Source: CAD feature listing. Evaluate the final solid. Frame: model axes, mm. Coordinates: 2 decimals unless noted, no trailing zeros. Order: outer loops, then holes, each group sorted by start corner. A loop starts at its lowest first (then second) coordinate and runs counter-clockwise, first axis right, second up.
Autodesk Inventor part; units mm, degrees
ref_plane "YZ Plane" through (0, 0, 0) normal (1, 0, 0) x (0, 1, 0)
ref_plane "XZ Plane" through (0, 0, 0) normal (0, 1, 0) x (-1, 0, 0)
ref_plane "XY Plane" through (0, 0, 0) normal (0, 0, 1) x (1, 0, 0)
sketch "Sketch1" plane through (0, 0, 0) normal (0, 0, 1) x (1, 0, 0)
  circle A0 centre (78.7027, 64.253) radius 50.8 construction
  circle A1 centre (-78.7027, -64.253) radius 50.8 construction
  circle A2 centre (0, 0) radius 50.8 construction
  line L0 (-39.3513, -32.1265) -> (39.3513, 32.1265) construction
  line L1 (78.7027, 64.253) -> (-78.7027, -64.253) construction
  line L2 (-3.7208, 6.6498) -> (-3.7208, 50.6636) construction
  line L3 (-410.4212, -115.053) -> (454.9708, -115.053) construction
  circle A3 centre (140.9799, -57.903) radius 57.15 construction
  circle A4 centre (78.7027, 64.253) radius 14.2621
  circle A5 centre (-78.7027, -64.253) radius 14.2621
  circle A6 centre (-3.7208, 6.6498) radius 57.15 construction
  circle A7 centre (-78.7027, -64.253) radius 30.1371 construction
  circle A8 centre (78.7027, 64.253) radius 30.1371 construction
  circle A9 centre (-45.946, 108.8074) radius 14.2621
  line L4 (-45.946, 108.8074) -> (78.7027, 64.253) construction
  circle A10 centre (78.7027, 64.253) radius 14.2875 construction
  circle A11 centre (-78.7027, -64.253) radius 14.2875 construction
  circle A12 centre (-70.3302, 67.854) radius 14.2621
  line L5 (-78.7027, -64.253) -> (-70.3302, 67.854) construction
  circle A13 centre (-70.3302, 67.854) radius 23.8316 construction
  circle A14 centre (-45.946, 108.8074) radius 23.8316 construction
  line L6 (20.6869, 58.3256) -> (65.8317, 37.0027)
  line L7 (-49.1354, -58.4201) -> (-59.7901, -4.4114)
  arc A15 (20.6869, 58.3256) -> (-59.7901, -4.4114) centre (-3.7208, 6.6498) ccw
  line L8 (-201.842, 171.7522) -> (-176.8279, 167.3416)
  line L9 (-176.8279, 167.3416) -> (-203.2918, 17.2569) construction
  line L10 (-203.2918, 17.2569) -> (-228.306, 21.6675) construction
  line L11 (-228.306, 21.6675) -> (-201.842, 171.7522) construction
  line L12 (-247.3095, -86.1068) -> (28.2095, -134.6882) construction
  line L13 (-202.9446, 165.4987) -> (190.461, 96.1307) construction
  line L14 (-202.9446, 165.4987) -> (-247.3095, -86.1068) construction
  circle A16 centre (-145.4023, 107.8713) radius 31.75 construction
  line L15 (-71.8375, 44.0702) -> (-75.4896, -13.5547) construction
  circle A17 centre (21.8974, 84.5575) radius 9.525 construction
  line L16 (-189.3349, 169.5469) -> (-215.7989, 19.4622) construction
  line L17 (-192.0916, 153.9131) -> (-213.0422, 35.096) construction
  circle A18 centre (-145.4023, 107.8713) radius 17.4625 construction
  circle A19 centre (-145.4023, 107.8713) radius 9.525
  circle A20 centre (-45.946, 108.8074) radius 30.1816 construction
  line L18 (-201.842, 171.7522) -> (-228.306, 21.6675)
  arc A21 (65.8317, 37.0027) -> (86.8534, 93.267) centre (78.7027, 64.253) ccw
  arc A22 (-108.4816, -68.8852) -> (-49.1354, -58.4201) centre (-78.7027, -64.253) ccw
  line L19 (-145.4023, 107.8713) -> (-128.993, 113.8438) construction
  line L20 (-111.0918, 120.3593) -> (-179.7129, 95.3833) construction
  circle A23 centre (-179.7129, 95.3833) radius 4.7625 construction
  line L21 (0, 0) -> (-3.7208, 6.6498) construction
  circle A24 centre (78.7027, 64.253) radius 28.6512 construction
  line L22 (66.1835, 38.4817) -> (-52.1778, 95.9789) construction
  line L23 (85.3564, 92.1209) -> (-42.6339, 122.6796) construction
  line L24 (-176.8279, 167.3416) -> (86.8534, 93.267)
  line L25 (-145.4023, 107.8713) -> (-121.2929, 36.7784) construction
  circle A25 centre (-121.2929, 36.7784) radius 31.75 construction
  circle A26 centre (-121.2929, 36.7784) radius 14.2621
  line L26 (-70.3302, 67.854) -> (-121.2929, 36.7784) construction
  circle A27 centre (-145.4023, 107.8713) radius 25.4 construction
  arc A28 (-108.4816, -68.8852) -> (-228.306, 21.6675) centre (-215.1488, -85.4777) ccw
  circle A29 centre (-145.4023, 107.8713) radius 36.5125 construction
  line L27 (-178.4939, 123.3021) -> (-145.4023, 107.8713) construction
  point P0 (-73.6635, 15.2577)
  point P1 (-202.5669, 94.5046)
  point P2 (-202.5669, 94.5046)
  point P3 (-142.37, 125.0685)
  point P4 (-158.7794, 119.096)
  point P5 (-161.8117, 101.8988)
  point P6 (-148.4347, 90.6741)
  point P7 (-132.0253, 96.6466)
  point P8 (-121.5341, 116.5586)
  point P9 (-140.9917, 132.8854)
  point P10 (-164.8599, 124.1981)
  point P11 (-169.2705, 99.184)
  point P12 (-149.813, 82.8572)
  point P13 (-125.9448, 91.5445)
  point P14 (-157.8903, 142.1818)
  point P15 (-179.7129, 95.3833)
  point P16 (-132.9143, 73.5608)
  point P17 (-129.9715, 140.9628)
  point P18 (-160.8332, 74.7797)
  point P19 (-112.3108, 92.4404)
  dimension "d7" = 101.6
  dimension "d18" = 47.6631
  dimension "d34" = 34.925
  dimension "d65" = 50.8
  dimension "d3" = 50.772
  dimension "d4" = 0
  dimension "d8" = 101.6
  dimension "d9" = 28.5242
  dimension "d10" = 101.6
  dimension "d11" = 114.3
  dimension "d12" = 114.3
  dimension "d13" = 15.875
  dimension "d14" = 15.875
  dimension "d15" = 132.3721
  dimension "d16" = 28.575
  dimension "d17" = 132.3721
  dimension "d19" = 47.6631
  dimension "d22" = 25.4
  dimension "d23" = 152.4
  dimension "d26" = 255.4869
  dimension "d27" = 63.5
  dimension "d30" = 203.2
  dimension "d31" = 10
  dimension "d32" = 19.05
  dimension "d33" = 120.65
  dimension "d35" = 19.05
  dimension "d36" = 6.35
  dimension "d40" = 360
  dimension "d44" = 9.525
  dimension "d55" = 80
  dimension "d56" = 7.62
  dimension "d58" = 57.3024
  dimension "d59" = 63.5
  dimension "d60" = 75.0697
  dimension "d61" = 59.69
  dimension "d62" = 55
  dimension "d68" = 360
  dimension "d70" = 41.275
  dimension "d71" = 60
  dimension "d82" = 360
  dimension "d87" = 360
  dimension "d89" = 45
  dimension "d90" = 6.35
  dimension "d91" = 20.955
  dimension "d92" = 107.95
extrude "Extrusion1" add sketch "Sketch1" along normal blind 6.35
hole "Hole1" at (21.8974, 84.5575, 0) at (-192.0916, 153.9131, 0) at (-202.5669, 94.5046, 0) at (-213.0422, 35.096, 0) at (-128.993, 113.8438, 0) at (-142.37, 125.0685, 0) at (-158.7794, 119.096, 0) at (-161.8117, 101.8988, 0) at (-148.4347, 90.6741, 0) at (-132.0253, 96.6466, 0) at (-111.0918, 120.3593, 0) at (-179.7129, 95.3833, 0) at (-149.813, 82.8572, 0) at (-169.2705, 99.184, 0) at (-164.8599, 124.1981, 0) at (-140.9917, 132.8854, 0) at (-121.5341, 116.5586, 0) at (-125.9448, 91.5445, 0) at (-73.6635, 15.2577, 0) at (-178.4939, 123.3021, 0) at (-129.9715, 140.9628, 0) at (-112.3108, 92.4404, 0) at (-160.8332, 74.7797, 0) direction (0, 0, 1) diameter 5.1054 end through all
sketch "Sketch2" plane through (0, 0, 6.35) normal (0, 0, 1) x (1, 0, 0)
  circle A0 centre (-125.9448, 91.5445) radius 2.5527 construction
  circle A1 centre (-140.9917, 132.8854) radius 2.5527 construction
  circle A2 centre (-169.2705, 99.184) radius 2.5527 construction
  circle A3 centre (-179.7129, 95.3833) radius 2.5527 construction
  circle A4 centre (-132.0253, 96.6466) radius 2.5527 construction
  circle A5 centre (-161.8117, 101.8988) radius 2.5527 construction
  circle A6 centre (-142.37, 125.0685) radius 2.5527 construction
  circle A7 centre (-213.0422, 35.096) radius 2.5527 construction
  circle A8 centre (-192.0916, 153.9131) radius 2.5527 construction
  circle A9 centre (21.8974, 84.5575) radius 2.5527 construction
  circle A10 centre (-202.5669, 94.5046) radius 2.5527 construction
  circle A11 centre (-128.993, 113.8438) radius 2.5527 construction
  circle A12 centre (-158.7794, 119.096) radius 2.5527 construction
  circle A13 centre (-148.4347, 90.6741) radius 2.5527 construction
  circle A14 centre (-111.0918, 120.3593) radius 2.5527 construction
  circle A15 centre (-149.813, 82.8572) radius 2.5527 construction
  circle A16 centre (-164.8599, 124.1981) radius 2.5527 construction
  circle A17 centre (-121.5341, 116.5586) radius 2.5527 construction
  circle A18 centre (-73.6635, 15.2577) radius 2.5527 construction
  line L0 (-49.1354, -58.4201) -> (-59.7901, -4.4114) construction
  arc A19 (20.6869, 58.3256) -> (-59.7901, -4.4114) centre (-3.7208, 6.6498) ccw construction
  line L1 (20.6869, 58.3256) -> (65.8317, 37.0027) construction
  arc A20 (65.8317, 37.0027) -> (86.8534, 93.267) centre (78.7027, 64.253) ccw construction
  line L2 (86.8534, 93.267) -> (-176.8279, 167.3416) construction
  line L3 (-176.8279, 167.3416) -> (-201.842, 171.7522) construction
  line L4 (-201.842, 171.7522) -> (-228.306, 21.6675) construction
  arc A21 (-108.4816, -68.8852) -> (-228.306, 21.6675) centre (-215.1488, -85.4777) ccw construction
  arc A22 (-108.4816, -68.8852) -> (-49.1354, -58.4201) centre (-78.7027, -64.253) ccw construction
  circle A23 centre (-70.3302, 67.854) radius 14.2621 construction
  circle A24 centre (-145.4023, 107.8713) radius 9.525 construction
  circle A25 centre (-121.2929, 36.7784) radius 14.2621 construction
  circle A26 centre (-45.946, 108.8074) radius 14.2621 construction
  circle A27 centre (-78.7027, -64.253) radius 14.2621 construction
  circle A28 centre (78.7027, 64.253) radius 14.2621 construction
  line L5 (-77.3732, -43.2766) -> (-80.0321, -85.2294) construction
  line L6 (-139.2383, 25.8358) -> (-103.3475, 47.721) construction
  line L7 (-69.0007, 88.8304) -> (-71.6596, 46.8776) construction
  line L8 (-65.7381, 115.8819) -> (-26.1538, 101.7329) construction
  line L9 (58.9105, 71.3275) -> (98.4948, 57.1785) construction
  circle A29 centre (-70.3302, 67.854) radius 14.2621 construction
  line L10 (-45.946, 108.8074) -> (-70.3302, 67.854) construction
  line L11 (-45.946, 108.8074) -> (78.7027, 64.253) construction
  line L12 (-70.3302, 67.854) -> (-121.2929, 36.7784) construction
  line L13 (-70.3302, 67.854) -> (-78.7027, -64.253) construction
  circle A30 centre (-112.3108, 92.4404) radius 2.5527
  point P0 (0, 0)
  point P1 (-116.0598, 70.5176)
  point P2 (-113.1961, 73.3575)
  dimension "d72" = 42.037
hole "Hole2" at (-77.3732, -43.2766, 6.35) at (-103.3475, 47.721, 6.35) at (-80.0321, -85.2294, 6.35) at (-139.2383, 25.8358, 6.35) at (-71.6596, 46.8776, 6.35) at (-69.0007, 88.8304, 6.35) at (-26.1538, 101.7329, 6.35) at (-65.7381, 115.8819, 6.35) at (98.4948, 57.1785, 6.35) at (58.9105, 71.3275, 6.35) direction (0, 0, -1) diameter 5.1054 end through all
properties part number "GP7-001" material "Polycarbonate, Smoke"
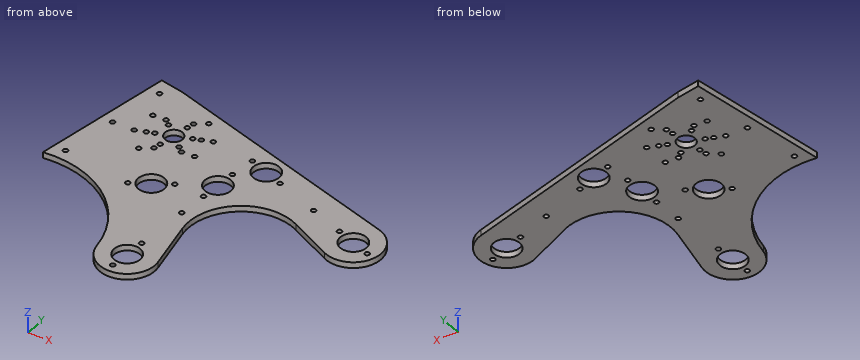
1. Ray query, line 1 (Y direction, x = -139.5, z = 2.25); line 2 (X direction, y = 46, z = 2.25); line 3 (Y direction, x = -144, z = 0.5). Return the intervals inside material, ascending.
Findings:
line 1: y = -8.47 to 23.3, 28.38 to 100.4, 115.35 to 130.81, 134.96 to 156.86
line 2: x = -224.02 to -132.17, -110.41 to -105.23, -101.46 to -74.06, -69.26 to -45.17, 46.78 to 102.68
line 3: y = -4.29 to 98.45, 117.29 to 123.1, 127.03 to 158.12
2. Pin query (flat end, axial travel): P1, Ø3, axis at x = -26.15, y = 101.73, coming from the -Z side; P2, Ø1, axis at y = -13, z = 3.5, coming from the -X side; P3, Ø1, axis at x = 20, z = 5, coming from the +Y side; P4, Ø3, axis at x = -177.5, z = 5, coming from the -Y side. Return the tip coordinate at first contact, or that it passes through.
Findings:
P1: passes through
P2: stops at x = -135.6
P3: stops at y = 112.19
P4: stops at y = 15.12
3. Section query B-B on y = -17. Return loops of the section in (x, z).
Findings:
outline: (-131.7, 0) - (-57.31, 0) - (-57.31, 6.35) - (-131.7, 6.35) - close
4. Section query C-C on x = -7. Return loops of the section in (y, z), plus the area to 3 significant figures.
Findings:
outline: (63.71, 0) - (119.63, 0) - (119.63, 6.35) - (63.71, 6.35) - close
area: 355 mm2
5. Section query A-A on z = 3. Count the separate pieces of the cut face and the enclosed holes in it, plus the area to 3 significant figures.
Findings:
separate pieces: 1
enclosed holes: 39
area: 35,200 mm2
